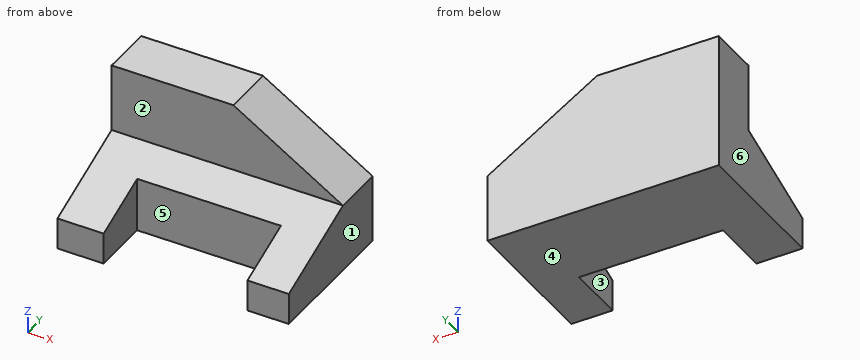
from build123d import *

# Parameters (mm, degrees)
F1_DEPTH = 95
F3_DEPTH = 21.2002830101
F5_DEPTH = 25
F6_W     = 59
F6_H     = 24
F7_DEPTH = 30


with BuildPart() as f1:
    # F0 (on Right) → F1 (new body)
    with BuildSketch(Plane.YZ):
        Polygon((-60, 0), (0, 0), (0, 56), (-21.2002830101, 56), (-21.2002830101, 28), (-60, 13), align=None)
    extrude(amount=-F1_DEPTH)

    # F2 (on face) → F3 (join, through all)
    with BuildSketch(Plane.XZ.offset(21.2002830101)):
        Polygon((0, 56), (-38.8899631798, 56), (0, 28), align=None)
    extrude(amount=-F3_DEPTH)

    # F4 (on face) → F5 (cut)
    with BuildSketch(Plane.XZ.offset(21.2002830101)):
        Polygon((0, 56), (-45, 56), (0, 28), align=None)
    extrude(amount=-F5_DEPTH, mode=Mode.SUBTRACT)

    # F6 (on face) → F7 (cut)
    with BuildSketch(Plane(origin=(0, 0, 0), x_dir=(1, 0, 0), z_dir=(0, 0, -1))):
        with Locations((-46.5, 48)):
            Rectangle(F6_W, F6_H)
    extrude(amount=-F7_DEPTH, mode=Mode.SUBTRACT)


with BuildPart() as f1_1:
    # F8: moved
    add(f1.part.moved(Location((95, 0, 0))))


solid = f1_1.part
Work out the finished part from the listing and answer in its coordinate system (mm). Face numbers are marked on the shaded views. A direction names the side the tool comes from. Round coordinates to 2 decimals unless told otherwise and drop trailing zeros. Write each loop counter-clockwise with the first axis right and the second up, starting at its lowest first coordinate (ties: lowest second). Pieces come first, ordered by that corner, then holes. Notation, with made-up numbers: (-39, 38.5) -> (-6, 38.5) arc R7 cw to (-6, 46.5) -> close; hole circle Ø2 at (14, 62.5). An arc over 180 degrees is marked (long way). Write each question's results on one line, items separated by ' | '.
Item 1: Find the intervals of material crossed by line 1 along X through (y, z) = (-54.5, 10.5); line 2 along Y through (x, z) = (32.5, 43); line 3 along Y through (x, z) = (36.5, 7.5), in increasing order. Write a range as [from, to].
Result set:
line 1: [0, 19], [78, 95] | line 2: [-21.2, 0] | line 3: [-36, 0]
Item 2: A cutting plane is placed at C-C, the plane y = -16. Determine the outline of the cut face in (x, z).
Result set:
outline: (0, 0) -> (95, 0) -> (95, 28) -> (50, 56) -> (0, 56) -> close
Item 3: A cutting plane is placed at B-B, the plane x = 23. Determine the outline of the cut face in (y, z).
Result set:
outline: (-36, 0) -> (0, 0) -> (0, 56) -> (-21.2, 56) -> (-21.2, 28) -> (-36, 22.28) -> close
Item 4: A cutting plane is placed at D-D, the plane z = 15. Determine the outline of the cut face in (x, y), plus the area to 3 significant figures.
Result set:
outline: (0, -54.83) -> (19, -54.83) -> (19, -36) -> (78, -36) -> (78, -54.83) -> (95, -54.83) -> (95, 0) -> (0, 0) -> close | area: 4,100 mm^2
Item 5: A cutting plane is placed at A-A, the plane y = -39.5. Determine the outline of the cut face in (x, z), plus the area to 3 significant figures.
Result set:
outline: (0, 0) -> (19, 0) -> (19, 20.93) -> (0, 20.93) -> close; (78, 0) -> (95, 0) -> (95, 20.93) -> (78, 20.93) -> close | area: 753 mm^2
Item 6: Which of the six approach directions +Z, -Z, +X, -X, +Y, -Y give full straight-line access (tool end or side, diameter ignored) to the marked faces 1, 2 and 3?
Result set:
face 1: +Z, -Z, +X, +Y, -Y | face 2: +Z, +X, -X, -Y | face 3: +Z, -Z, -Y
Item 7: Flat-ended cylindrical pins translate along their axes: P1, Ø12, axis at x = 64, y = -22.5, coming from the +Z side; P2, Ø1, axis at x = 21.5, z = 29, coming from the -Y side; P3, Ø6.5, axis at x = 44.5, z = 10, coming from the -Y side. Find the tip coordinate at first contact, or state that the pin passes through.
Result set:
P1: z = 50.93 | P2: y = -21.2 | P3: y = -36
Item 8: The mould has two halves that part along X. Classify the marked faces 4, 5 and 6: +X half, -X half, draft (parallel to the pull), parting line (faces both ways), or undercut.
Result set:
face 4: draft | face 5: undercut | face 6: -X half
